Source: CAD feature listing. Evaluate the final solid. Frame: model axes, mm. Give positions to 0.01 mm unless a question says otherwise; leave off trailing zeros. Loops run counter-clockwise (first coordinate to the right, second up) from the corner with the lowest first, then second, coordinate; pieces in that order, holes last. Notation, with made-up numbers: (-38, -19) -> (-32, -19) arc R20 cw to (-32, 17) -> close; hole circle Ø9 at (-8.75, -19.5). An arc over 180 degrees is marked (long way). Return JSON: item names as keys, results as strings. Group by question number.
(1) Cut plane A-A on z = 56. Return loops of the section in (x, y), then the cut area to 3 significant figures.
(2) Cut plane B-B on x = 6. Return loops of the section in (y, z).
(3) Cut plane D-D on y = 0.65. Give the number of separate pieces and of enclosed holes in the cut face, then the cut area to 3 significant figures.
(4) Ray query, line 1 (X direction, y = 1.95, z = 56); line 2 (X direction, y = 1.3, z = -40); line 3 (Z direction, x = -20, y = 0.95). Return the intervals inside material, ascending. Write a range as from..to.
(5) Cut plane C-C on x = -81. Return loops of the section in (y, z).
(6) Pin query (flat end, axial travel): pin 1 (1.2 mm diameter, centred on x = 98.5, y = 1.5, fed in from +Z); pin 2 (2 mm diameter, centred on y = 2, z = 73.5, fed in from -X). Return the tip coordinate at first contact, or that it passes through.
```python
from build123d import *

# Parameters (mm, degrees)
ESBO_O1_W                               = 200
ESBO_O1_H                               = 150
RESSALTO_EXTRUS_O1_DEPTH                = 4
ESBO_O2_W                               = 35
ESBO_O2_H                               = 4
ESBO_O2_W_2                             = 4
ESBO_O2_H_2                             = 30
CORTE_EXTRUS_O1_DEPTH                   = 5
ESBO_O3_W                               = 200
ESBO_O3_H                               = 15
CORTE_EXTRUS_O2_DEPTH                   = 5
BROCA_DE_ROSQUEAR_PARA_TARRAXA_DE_M41_D = 4.5
ESBO_O5_R                               = 2.25
CORTE_EXTRUS_O3_DEPTH                   = 5


with BuildPart() as part:
    # Esboço1 → Ressalto-extrusão1 (new body)
    with BuildSketch(Plane(origin=(0, 0, 0), x_dir=(1, 0, 0), z_dir=(0, 1, 0))):
        Rectangle(ESBO_O1_W, ESBO_O1_H)
    extrude(amount=RESSALTO_EXTRUS_O1_DEPTH)

    # Esboço2 → Corte-extrusão1 (cut, through all)
    with BuildSketch(Plane(origin=(0, 4, 0), x_dir=(1, 0, 0), z_dir=(0, 1, 0))):
        with Locations((-27.5, -73)):
            Rectangle(ESBO_O2_W, ESBO_O2_H)
        with Locations((27.5, -73)):
            Rectangle(ESBO_O2_W, ESBO_O2_H)
        with Locations((82.5, -73)):
            Rectangle(ESBO_O2_W, ESBO_O2_H)
        with Locations((-82.5, -73)):
            Rectangle(ESBO_O2_W, ESBO_O2_H)
        with Locations((98, 30)):
            Rectangle(ESBO_O2_W_2, ESBO_O2_H_2)
        with Locations((98, -30)):
            Rectangle(ESBO_O2_W_2, ESBO_O2_H_2)
        with Locations((-98, 30)):
            Rectangle(ESBO_O2_W_2, ESBO_O2_H_2)
        with Locations((-98, -30)):
            Rectangle(ESBO_O2_W_2, ESBO_O2_H_2)
    extrude(amount=-CORTE_EXTRUS_O1_DEPTH, mode=Mode.SUBTRACT)

    # Esboço3 → Corte-extrusão2 (cut, through all)
    with BuildSketch(Plane(origin=(0, 4, 0), x_dir=(1, 0, 0), z_dir=(0, 1, 0))):
        with Locations((0, 67.5)):
            Rectangle(ESBO_O3_W, ESBO_O3_H)
    extrude(amount=-CORTE_EXTRUS_O2_DEPTH, mode=Mode.SUBTRACT)

    # Broca de rosquear para tarraxa de M41 (through all)
    with Locations(Plane(origin=(-81, 4, -40), x_dir=(0, 0, 1), z_dir=(0, 1, 0))):
        with Locations((0, 0), (96, 0), (96, 162), (0, 162)):
            Hole(BROCA_DE_ROSQUEAR_PARA_TARRAXA_DE_M41_D / 2)

    # Esboço5 → Corte-extrusão3 (cut, through all)
    with BuildSketch(Plane(origin=(0, 4, 0), x_dir=(1, 0, 0), z_dir=(0, 1, 0))):
        with Locations((-81, -56)):
            Circle(ESBO_O5_R)
        with BuildLine():
            Line((55, -61), (-55, -61))
            ThreePointArc((-55, -61), (-60, -56), (-55, -51))
            Line((-55, -51), (55, -51))
            ThreePointArc((55, -51), (60, -56), (55, -61))
        make_face()
    extrude(amount=-CORTE_EXTRUS_O3_DEPTH, mode=Mode.SUBTRACT)


solid = part.part
```
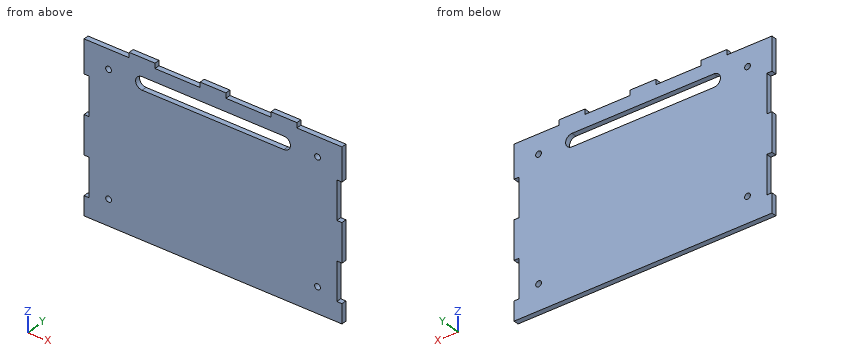
Answers:
{
 "1": {"outline": "(-100, 0) -> (-83.25, 0) -> (-83.25, 4) -> (-100, 4) -> close; (-78.75, 0) -> (-60, 0) -> (-60, 4) -> (-78.75, 4) -> close; (60, 0) -> (78.75, 0) -> (78.75, 4) -> (60, 4) -> close; (83.25, 0) -> (100, 0) -> (100, 4) -> (83.25, 4) -> close", "area": "284 mm²"},
 "2": {"outline": "(0, -60) -> (4, -60) -> (4, 51) -> (0, 51) -> close; (0, 61) -> (4, 61) -> (4, 75) -> (0, 75) -> close"},
 "3": {"separate pieces": "1", "enclosed holes": "5", "area": "24,700 mm²"},
 "4": {"line 1": "-100..-83.25, -78.75..-60, 60..78.75, 83.25..100", "line 2": "-96..-83.25, -78.75..78.75, 83.25..96", "line 3": "-60..51, 61..71"},
 "5": {"outline": "(0, -60) -> (4, -60) -> (4, -42.25) -> (0, -42.25) -> close; (0, -37.75) -> (4, -37.75) -> (4, 53.75) -> (0, 53.75) -> close; (0, 58.25) -> (4, 58.25) -> (4, 71) -> (0, 71) -> close"},
 "6": {"pin 1": "z = 71", "pin 2": "x = -65"}
}
